```python
from build123d import *

# Parameters (mm, degrees)
F1_DEPTH = 30
F2_R     = 2.55
F3_DEPTH = 6
F2_R_2   = 4
F4_DEPTH = 2


with BuildPart() as f1:
    # F0 (on Top) → F1 (new body)
    with BuildSketch(Plane.XY):
        with BuildLine():
            Line((-34, 5), (-34, 0))
            Line((-34, 0), (-14.5688022843, 0))
            ThreePointArc((-14.5688022843, 0), (-16.37669445, 2.3759309202), (-17.8006970079, 5))
            Line((-17.8006970079, 5), (-34, 5))
        make_face()
        with BuildLine():
            ThreePointArc((-17.8006970079, 5), (-16.37669445, 2.3759309202), (-14.5688022843, 0))
            Line((-14.5688022843, 0), (-12.1187793927, 0))
            Line((-12.1187793927, 0), (-12.1187793927, 5))
            Line((-12.1187793927, 5), (-17.8006970079, 5))
        make_face()
        with BuildLine():
            ThreePointArc((19.5, 12.9614813968), (-4.0704058978, 32.0319243866), (-17.8006970079, 5))
            Line((-17.8006970079, 5), (-12.1187793927, 5))
            ThreePointArc((-12.1187793927, 5), (-4.1549788692, 26.8534269264), (14.5, 12.9614813968))
            ThreePointArc((14.5, 12.9614813968), (13.8919455296, 8.8065025277), (12.1187793927, 5))
            Line((12.1187793927, 5), (17.8006970079, 5))
            ThreePointArc((17.8006970079, 5), (19.0704429898, 8.891075499), (19.5, 12.9614813968))
        make_face()
        with BuildLine():
            Line((12.1187793927, 0), (14.5688022843, 0))
            ThreePointArc((14.5688022843, 0), (16.37669445, 2.3759309202), (17.8006970079, 5))
            Line((17.8006970079, 5), (12.1187793927, 5))
            Line((12.1187793927, 5), (12.1187793927, 0))
        make_face()
        with BuildLine():
            ThreePointArc((17.8006970079, 5), (16.37669445, 2.3759309202), (14.5688022843, 0))
            Line((14.5688022843, 0), (34, 0))
            Line((34, 0), (34, 5))
            Line((34, 5), (17.8006970079, 5))
        make_face()
    extrude(amount=F1_DEPTH)

    # F2 (on face) → F3 (cut)
    with BuildSketch(Plane(origin=(0, 5, 0), x_dir=(-1, 0, 0), z_dir=(0, 1, 0))):
        with Locations((-24.75, 15)):
            Circle(F2_R)
        with Locations((24.75, 15)):
            Circle(F2_R)
    extrude(amount=-F3_DEPTH, mode=Mode.SUBTRACT)

    # F2 (on face) → F4 (cut)
    with BuildSketch(Plane(origin=(0, 5, 0), x_dir=(-1, 0, 0), z_dir=(0, 1, 0))):
        with Locations((24.75, 15)):
            Circle(F2_R_2)
        with Locations((24.75, 15)):
            Circle(F2_R, mode=Mode.SUBTRACT)
        with Locations((-24.75, 15)):
            Circle(F2_R_2)
        with Locations((-24.75, 15)):
            Circle(F2_R, mode=Mode.SUBTRACT)
    extrude(amount=-F4_DEPTH, mode=Mode.SUBTRACT)


solid = f1.part
```
Verification items for the finished model (mm, model axes). A direction names the side the tool comes from. Give positions to 0.01 mm unless a question says otherwise; leave off trailing zeros. Loops run counter-clockwise (first coordinate to the right, second up) from the corner with the lowest first, then second, coordinate; pieces in that order, holes last. Notation, with made-up numbers: M -16.75,-19.75 L 31.25,-19.75 A12 cw 31.25,-0.75 Z; hole C 45.5,-32.75 d4. An arc over 180 degrees is marked long. Return JSON: item names as keys, results as strings.
1) Section check A-A, the plane z = 15. Enter the section's corners in (x, y).
Findings:
{"outline": "M -34,0 L -27.3,0 L -27.3,3 L -28.75,3 L -28.75,5 L -34,5 Z; M -22.2,0 L -12.12,0 L -12.12,5 A14.5 cw long 12.12,5 L 12.12,0 L 22.2,0 L 22.2,3 L 20.75,3 L 20.75,5 L 17.8,5 A19.5 ccw long -17.8,5 L -20.75,5 L -20.75,3 L -22.2,3 Z; M 27.3,0 L 34,0 L 34,5 L 28.75,5 L 28.75,3 L 27.3,3 Z"}
2) Section check D-D, the plane z = 23. Enter the section's corners in (x, y).
Findings:
{"outline": "M -34,0 L -12.12,0 L -12.12,5 A14.5 cw long 12.12,5 L 12.12,0 L 34,0 L 34,5 L 17.8,5 A19.5 ccw long -17.8,5 L -34,5 Z"}
3) Section check B-B, the plane x = 24.75. Enter the section's corners in (y, z).
Findings:
{"outline": "M 0,0 L 5,0 L 5,11 L 3,11 L 3,12.45 L 0,12.45 Z; M 0,17.55 L 3,17.55 L 3,19 L 5,19 L 5,30 L 0,30 Z"}
4) Mould release check, pull along Z, two halves, no side actions. Record for faces 1 (the flat face through (-13, 20, 30)), 2 (the cylindrical face through (-22.726, 1.521, 13.448)), 3 (the flat face through (12.119, 3, 15)): released by +Z, released by -Z, zero draft, split by the parting line, or undercut.
Findings:
{"face 1": "released by +Z", "face 2": "undercut", "face 3": "zero draft"}
5) Tool access check on faces 4 (the flat face through (20, 0, 15)), 5 (the flat face through (-29, 5, 15)), 6 (the flat face through (22, 3, 15)), 7 (the flat face through (-12.119, 2, 15)), 8 (the flat face through (30, 5, 15)). Record the directions out of +Z, -Z, +X, -X, +Y, -Y that give a thin tool (end or side, any length) a straight path to the whole face; none if there is none.
Findings:
{"face 4": "+Z, -Z, +X, -X, -Y", "face 5": "+Z, -Z, -X", "face 6": "+Y", "face 7": "+Z, -Z, -Y", "face 8": "+Z, -Z, +X"}
6) Gauge pin test, flat ends, axial feed: P1, Ø5, axis at y = 9, z = 21.5, coming from the -X side; P2, Ø6, axis at y = 22, z = 14, coming from the +X side; P3, Ø9, axis at x = 24.5, z = 16.5, coming from the +Y side. Record the tip position at first contact, or that the pin passes through.
Findings:
{"P1": "stops at x = -19.45", "P2": "stops at x = 18.54", "P3": "stops at y = 5"}
7) Section check C-C, the plane y = 25. Enter the section's corners in (x, z).
Findings:
{"outline": "M -15.34,0 L -8.08,0 L -8.08,30 L -15.34,30 Z; M 8.08,0 L 15.34,0 L 15.34,30 L 8.08,30 Z"}
8) Material ranges on L1, parallel to Z at x = -24.75, y = 0.65; L2, parallel to Y at x = 27.5, z = 26.5; L3, parallel to Z at x = -24.75, y = 4, recorded low to high. Write a range as [from, to].
Findings:
{"L1": "z = [0, 12.45], [17.55, 30]", "L2": "y = [0, 5]", "L3": "z = [0, 11], [19, 30]"}
